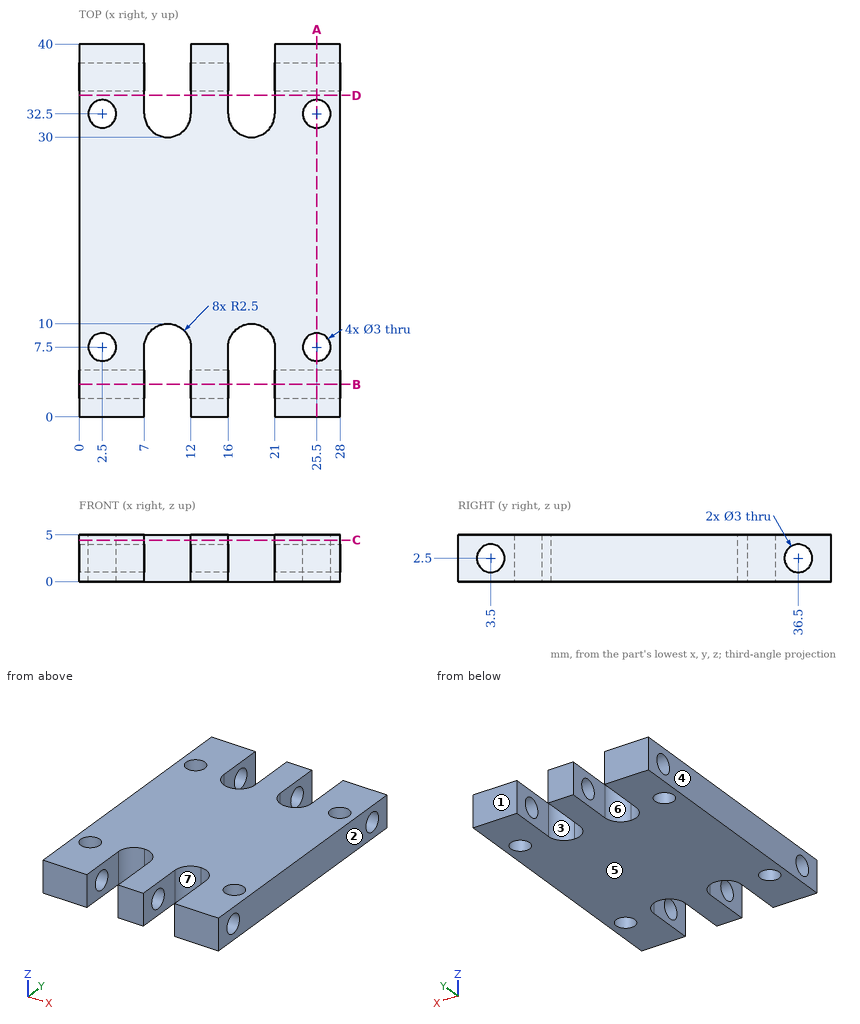
Job drawing, mm, ordinate dimensions from the low corner. One solid piece. A direction names the side the tool comes from. Give positions to 0.01 mm unless a question says otherwise; leave off trailing zeros. Write each loop counter-clockwise with the first axis right and the second up, starting at its lowest first coordinate (ties: lowest second). Pieces come first, ordered by that corner, then holes. Notation, with made-up numbers: M 63,-4.75 L 71,-4.75 A31 cw 71,23.25 Z; hole C 32,17.25 d9. An arc over 180 degrees is marked long. Put each result on its own line as item: value. Start each with the question number.
(1) Band-saw the part on A-A, the plane x = 25.5. Write the cut outline in (y, z), and give its area (3 significant figures).
(2) Which spindle directions (+Z, -Z, +X, -X, +Y, -Y) get a long thin tool onto all of the face, cutting with end or side? Do the marked faces 5, 6 and 7. Say none if no direction does.
(3) Band-saw the part on C-C, the plane z = 4.45. Give the number of separate pieces and of enclosed holes in the cut face.
(4) Flat gauge pins, fed straight in: pin 1 Ø1 at (x, z) = (8.5, 3.5) entering from -Y; pin 2 Ø1.8 at (y, z) = (36.5, 2.5) entering from -X (1 decimal). Where does each tip first touch, or does it go through?
(5) Band-saw the part on B-B, the plane y = 3.5. Write the cut outline in (x, z), and give its area (3 significant figures).
(6) Mould opens along X. For the marked faces 1, 2, 3 and 4 say: +X half, -X half, draft (parallel to the pull), parting line (faces both ways), or undercut.
(7) Band-saw the part on D-D, the plane y = 34.5. Write the cut outline in (x, z), and give its area (3 significant figures).
(8) Probe L1, parallel to X at y = 37, z = 4.35; L2, parallel to Z at x = 14.1, y = 3.5; L3, parallel to X at y = 33.5, z = 3.7. List the from-to ranges inside material, lowest first.
Response values:
1. outline: M 0,0 L 6,0 L 6,5 L 0,5 Z; M 9,0 L 31,0 L 31,5 L 9,5 Z; M 34,0 L 40,0 L 40,5 L 34,5 Z; hole C 3.5,2.5 d3; hole C 36.5,2.5 d3
1. area: 156 mm2
2. face 5: -Z, +X, -X, +Y, -Y
2. face 6: +Z, -Z, +Y
2. face 7: +Z, -Z, -Y
3. separate pieces: 1
3. enclosed holes: 4
4. pin 1: stops at y = 9.5
4. pin 2: passes through
5. outline: M 0,0 L 7,0 L 7,1 L 0,1 Z; M 0,4 L 7,4 L 7,5 L 0,5 Z; M 12,0 L 16,0 L 16,1 L 12,1 Z; M 12,4 L 16,4 L 16,5 L 12,5 Z; M 21,0 L 28,0 L 28,1 L 21,1 Z; M 21,4 L 28,4 L 28,5 L 21,5 Z
5. area: 36.0 mm2
6. face 1: draft
6. face 2: +X half
6. face 3: undercut
6. face 4: -X half
7. outline: M 0,0 L 7,0 L 7,5 L 0,5 Z; M 12,0 L 16,0 L 16,5 L 12,5 Z; M 21,0 L 28,0 L 28,5 L 21,5 Z
7. area: 90.0 mm2
8. L1: x = 0 to 7, 12 to 16, 21 to 28
8. L2: z = 0 to 1, 4 to 5
8. L3: x = 0 to 1.38, 3.62 to 7, 12 to 16, 21 to 24.38, 26.62 to 28
